The listing builds one solid part. Answer for the finished solid, in the listing's coordinates (mm). Face numbers are marked on the shaded views. A direction names the side the tool comes from. Round coordinates to 2 decimals unless told otherwise and drop trailing zeros. Loops run counter-clockwise (first coordinate to the right, second up) from the corner with the lowest first, then second, coordinate; pieces in that order, holes last. Notation, with made-up numbers: (43.5, 28.25) - (57.5, 28.25) arc R34 cw to (57.5, 61.25) - close; hole circle Ø9 at (17, 76.25). An arc over 180 degrees is marked (long way). One line per item, written item: value.
Autodesk Inventor part; units mm, degrees
ref_plane "Work Plane1" through (0, 0, 10) normal (0, 0, 1) x (1, 0, 0)
ref_plane "Work Plane2" through (0, -18.5, 17.5) normal (0, -1, 0) x (1, 0, 0)
ref_plane "Work Plane3" through (-7.5, 0, 25) normal (0, -1, 0) x (1, 0, 0)
sketch "Sketch2" plane through (0, 0, 0) normal (0, 0, 1) x (1, 0, 0)
  circle A0 centre (0, 0) radius 7.5
  dimension "d1" = 15
ref_plane "Work Plane1" through (0, 0, 10) normal (0, 0, 1) x (1, 0, 0)
sketch "Sketch3" plane through (0, 0, 10) normal (0, 0, 1) x (1, 0, 0)
  line L0 (-7.5, -7.5) -> (7.5, -7.5)
  line L1 (7.5, -7.5) -> (7.5, 7.5)
  line L2 (7.5, 7.5) -> (-7.5, 7.5)
  line L3 (-7.5, 7.5) -> (-7.5, -7.5)
  line L4 (-7.5, -7.5) -> (7.5, 7.5) construction
  line L5 (7.5, -7.5) -> (-7.5, 7.5) construction
  point P0 (0, 0)
  dimension "d5" = 15
  dimension "d6" = 15
loft "Loft1" add profiles "Sketch2", "Sketch3"
sketch "Sketch4" plane through (-7.5, -7.5, 10) normal (0, 0, 1) x (1, 0, 0)
  line L0 (12.8033, 12.8033) -> (15, 15)
  line L1 (0, 0) -> (15, 0)
  line L2 (15, 0) -> (15, 15)
  line L3 (15, 15) -> (0, 15)
  line L4 (0, 15) -> (0, 0)
  line L5 (0, 0) -> (15, 15) construction
  line L6 (15, 0) -> (0, 15) construction
  point P0 (7.5, 7.5)
  dimension "d11" = 15
  dimension "d12" = 15
extrude "Extrusion2" add sketch "Sketch4" along normal blind 15
sketch "Sketch5" plane through (-7.5, -7.5, 25) normal (0, -1, 0) x (1, 0, 0)
  circle A0 centre (7.5, -7.5) radius 6.5
  point P0 (7.5, -25)
  point P1 (15, -15)
  dimension "d15" = 13
extrude "Extrusion3" add sketch "Sketch5" along normal blind 5
sketch "Sketch6" plane through (0, -12.5, 17.5) normal (0, -1, 0) x (1, 0, 0)
  circle A0 centre (0, 0) radius 7.5
  point P0 (0, -17.5)
  dimension "d24" = 15
ref_plane "Work Plane2" through (0, -18.5, 17.5) normal (0, -1, 0) x (1, 0, 0)
sketch "Sketch7" plane through (0, -18.5, 17.5) normal (0, -1, 0) x (1, 0, 0)
  circle A0 centre (0, 0) radius 6.5
  point P0 (0, -17.5)
loft "Loft2" add profiles "Sketch6", "Sketch7"
fillet "Fillet1" radius 2 1 edges at (-6.5, -12.5, 17.5)
fillet "Fillet2" radius 3 1 edges at (-6.5, -18.5, 17.5)
fillet "Fillet3" radius 5 1 edges at (-7.5, -12.5, 17.5)
ref_plane "Work Plane3" through (-7.5, 0, 25) normal (0, -1, 0) x (1, 0, 0)
mirror "Mirror1" about plane through (-7.5, 0, 25) normal (0, -1, 0) of "Fillet2", "Loft2", "Fillet3", "Fillet1", "Extrusion3"
fillet "Fillet4" radius 7.25 4 edges at (-7.5, 0, 25) (0, 7.5, 25) (7.5, 0, 25) (0, -7.5, 25)
properties part number "Palu"
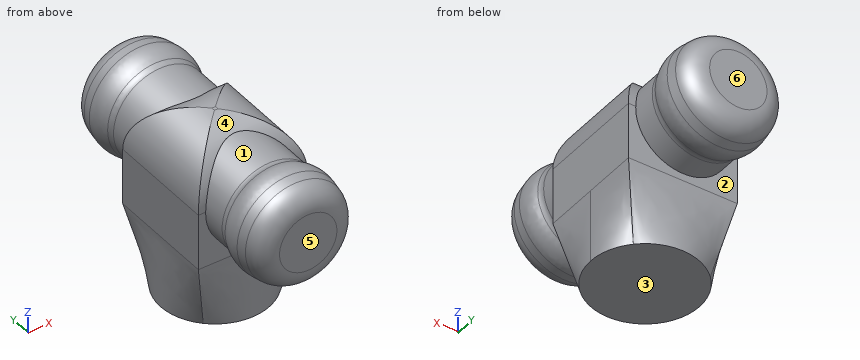
1) A cutting plane is placed at A-A on y = 15.5. Give the vertices of the cut face in (x, z).
Final values:
outline: circle Ø14 at (0, 17.5)
2) Consider L1, parallel to Y at x = -5.5, z = 11.25; L2, parallel to X at y = 0, z = 19.75; L3, parallel to Y at x = -5.25, z = 19.5. Determine where each line is inside the solid, lowest interval first.
Final values:
L1: -7.5 to 7.5
L2: -7.22 to 7.22
L3: -18 to 18
3) For a pull along Y with two mould halves and no side action, classify the marked faces 4, 5 and 6 as released by +Y, released by -Y, zero draft, split by the parting line, or undercut.
Final values:
face 4: undercut
face 5: released by -Y
face 6: released by +Y
4) Each of these flat-tipped pins is pushed along its axis until it touches: pin 1 Ø1 at (x, y) = (-2.5, -12.5) entering from +Z; pin 2 Ø1 at (y, z) = (-0.5, 19.5) entering from +X; pin 3 Ø10 at (y, z) = (-13, 9.5) entering from +X. Where does it stop, or does it pass through?
Final values:
pin 1: z = 24.28
pin 2: x = 7.39
pin 3: x = 6.53
5) For the marked faces 1, 2 and 3, determine the directions among +Z, -Z, +X, -X, +Y, -Y from which every point of the face is accessible in a straight line to the end or side of a thin tool.
Final values:
face 1: none
face 2: -Z
face 3: -Z, +X, -X, +Y, -Y
